```python
from build123d import *

# Parameters (mm, degrees)
SKETCH1_W           = 60.900023998
SKETCH1_H           = 150.828343314
SKETCH1_R           = 20.618232522
SKETCH1_W_2         = 47.971880286
SKETCH1_H_2         = 16.806586826
BOSS_EXTRUDE1_DEPTH = 63.5
SKETCH2_R           = 5.382285962
SKETCH2_R_2         = 4.862937902
BOSS_EXTRUDE2_DEPTH = 5


with BuildPart() as part:
    # Sketch1 → Boss-Extrude1 (new body)
    with BuildSketch(Plane.XY):
        Rectangle(SKETCH1_W, SKETCH1_H)
        Circle(SKETCH1_R, mode=Mode.SUBTRACT)
        with Locations((0, -57.530239521)):
            Rectangle(SKETCH1_W_2, SKETCH1_H_2, mode=Mode.SUBTRACT)
        with Locations((0, 57.530239521)):
            Rectangle(SKETCH1_W_2, SKETCH1_H_2, mode=Mode.SUBTRACT)
    extrude(amount=BOSS_EXTRUDE1_DEPTH)

    # Sketch2 → Boss-Extrude2 (add)
    with BuildSketch(Plane(origin=(0, 0, 0), x_dir=(-1, 0, 0), z_dir=(0, 0, -1))):
        Polygon((30.450011999, 93.405223195), (30.450011999, 75.414171657), (30.450011999, 0), (49.048404874, 0), (49.048404874, 93.405223195), align=None)
        with Locations((38.598962097, 34.973645215)):
            Circle(SKETCH2_R, mode=Mode.SUBTRACT)
        with Locations((38.598962097, 81.676256812)):
            Circle(SKETCH2_R_2, mode=Mode.SUBTRACT)
    extrude(amount=-BOSS_EXTRUDE2_DEPTH)


solid = part.part
```
Check sheet for the modelled part. Datum: model origin and axes. Units: mm. A direction names the side the tool comes from. Coordinates: 2 decimals unless noted, no trailing zeros. Order: outer loops, then holes, each group sorted by start corner. A loop starts at its lowest first (then second) coordinate and runs counter-clockwise, first axis right, second up. Notation, with made-up numbers: M 11.5,63.25 L 55.5,63.25 A23 cw 55.5,96.25 Z; hole C 76,73 d4. An arc over 180 degrees is marked long. Write each question's results on one line, items separated by ' | '. Start each with the question number.
1. Cross-section at A-A on y = 80. Record the cut outline in (x, z), and give its area (3 significant figures).
2. Cross-section at B-B on x = 0. Record the cut outline in (y, z).
3. Mould release check, pull along Y, two halves, no side actions. Record for faces 1 (the face through (-30.45, 85, 2)), 2 (the face through (-37.43, 29.72, 2.46)), 3 (the face through (-40, 0, 2)), 4 (the face through (23.986, -58, 31)): +Y half, -Y half, draft (parallel to the pull), parting line (faces both ways), or undercut.
4. Material ranges on probe 1 along Y at (x, z) = (0, 23); probe 2 along Y at (x, z) = (-21.5, 35.5); probe 3 along Y at (x, z) = (-18, 49.5), recorded low to high.
5. Cross-section at D-D on y = 28. Record the cut outline in (x, z), and give its area (3 significant figures).
6. Go/stop test with flat-tipped pins: P1, Ø3, axis at x = -12.5, z = 16.5, coming from the +Y side; P2, Ø13.5, axis at y = 61, z = 27, coming from the -X side; P3, Ø9.5, axis at x = -44, y = 54, coming from the +Z side; P4, Ø6, axis at x = -38.6, y = 81.68, coming from the -Z side. Record where each tip stops, or that it passes through.
7. Access from +Z, -Z, +X, -X, +Y, -Y to the whole of each face (thin tool, end or side, straight path). Record for faces 5 (the face through (-21, 1, 63.5)), 6 (the face through (-40, 47, 5)), 7 (the face through (0, 65.934, 31)).
8. Cross-section at C-C on z = 42. Record the cut outline in (x, y).
Checks:
1) outline: M -49.05,0 L -43.16,0 L -43.16,5 L -49.05,5 Z; M -34.03,0 L -30.45,0 L -30.45,5 L -34.03,5 Z | area: 47.3 mm²
2) outline: M -75.41,0 L -65.93,0 L -65.93,63.5 L -75.41,63.5 Z; M -49.13,0 L -20.62,0 L -20.62,63.5 L -49.13,63.5 Z; M 20.62,0 L 49.13,0 L 49.13,63.5 L 20.62,63.5 Z; M 65.93,0 L 75.41,0 L 75.41,63.5 L 65.93,63.5 Z
3) face 1: draft | face 2: undercut | face 3: -Y half | face 4: undercut
4) probe 1: y = -75.41 to -65.93, -49.13 to -20.62, 20.62 to 49.13, 65.93 to 75.41 | probe 2: y = -75.41 to -65.93, -49.13 to 49.13, 65.93 to 75.41 | probe 3: y = -75.41 to -65.93, -49.13 to -10.06, 10.06 to 49.13, 65.93 to 75.41
5) outline: M -49.05,0 L 30.45,0 L 30.45,63.5 L -30.45,63.5 L -30.45,5 L -49.05,5 Z | area: 3,960 mm²
6) P1: stops at y = 75.41 | P2: stops at x = -30.45 | P3: stops at z = 5 | P4: passes through
7) face 5: +Z, +X, -X, +Y, -Y | face 6: +Z, -X, +Y, -Y | face 7: +Z, -Z
8) outline: M -30.45,-75.41 L 30.45,-75.41 L 30.45,75.41 L -30.45,75.41 Z; hole M -23.99,-65.93 L 23.99,-65.93 L 23.99,-49.13 L -23.99,-49.13 Z; hole M -23.99,49.13 L 23.99,49.13 L 23.99,65.93 L -23.99,65.93 Z; hole C 0,0 d41.24
